Read the model definition and answer for the solid it produces. Units are mm, in the model's axes. Face numbers are marked on the shaded views. A direction names the side the tool comes from. Coordinates: 2 decimals unless noted, no trailing zeros. Write each loop counter-clockwise with the first axis right and the second up, starting at its lowest first coordinate (ties: lowest second). Pieces come first, ordered by that corner, then holes.
from build123d import *

# Parameters (mm, degrees)
CROQUIS1_R              = 11
CROQUIS3_R              = 11.5
CROQUIS4_R              = 7.5
CROQUIS5_R              = 8
CROQUIS6_R              = 16
CROQUIS6_R_2            = 8
SALIENTE_EXTRUIR1_DEPTH = 2


with BuildPart() as part:
    # Croquis1 → Recubrir1 section 0
    with BuildSketch(Plane.XY):
        Circle(CROQUIS1_R)
    # Croquis3 → Recubrir1 section 1
    with BuildSketch(Plane.XY.offset(33)):
        Circle(CROQUIS3_R)
    loft()

    # Croquis4 → Cortar-Recubrir1 section 0
    with BuildSketch(Plane(origin=(0, 0, 0), x_dir=(-1, 0, 0), z_dir=(0, 0, -1))):
        Circle(CROQUIS4_R)
    # Croquis5 → Cortar-Recubrir1 section 1
    with BuildSketch(Plane.XY.offset(33)):
        Circle(CROQUIS5_R)
    loft(mode=Mode.SUBTRACT)

    # Croquis6 → Saliente-Extruir1 (add)
    with BuildSketch(Plane.XY.offset(33)):
        Circle(CROQUIS6_R)
        Circle(CROQUIS6_R_2, mode=Mode.SUBTRACT)
    extrude(amount=SALIENTE_EXTRUIR1_DEPTH)


solid = part.part
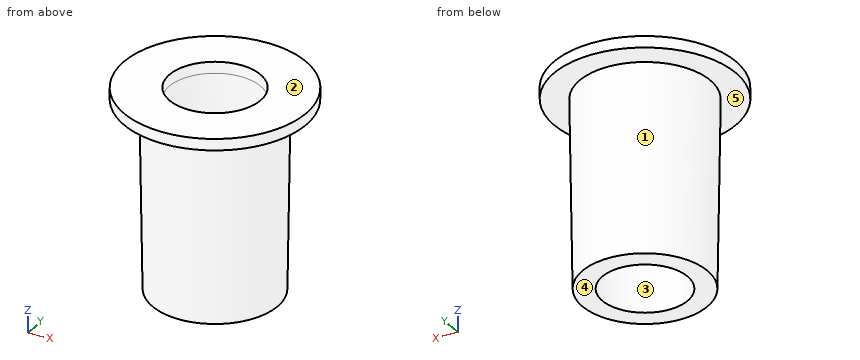
Item 1: The part is cut by section A-A (z = 14). Give the vertices of the cut face in (x, y).
Item 2: Find the intervals of material crossed by probe 1 along Y at (x, z) = (0, 34.5); probe 2 along Y at (x, z) = (-7, 25); probe 3 along X at (y, z) = (6, 10.5), in increasing order.
Item 3: Given pin 1 (2 mm diameter, centred on y = 12.5, z = 20.5, fed in from -X); pin 2 (5 mm diameter, centred on y = 7, z = 15, fed in from -X); pin 3 (4 mm diameter, centred on y = -10.5, z = 18, fed in from +X), each flat-ended and moving along its own axis, determine where each tip first touches the part or whether it passes through.
Item 4: For the marked faces 4 and 5, determine the directions among +Z, -Z, +X, -X, +Y, -Y from which every point of the face is accessible in a straight line to the end or side of a thin tool.
Item 5: The part is cut by section C-C (z = 9.5). Give the vertices of the cut face in (x, y).
Item 6: Determine the mould class of the marked faces 1, 2 and 3 for opening direction X: +X half, -X half, draft (parallel to the pull), parting line (faces both ways), or undercut.
Item 7: The part is cut by section B-B (x = 13.5). Give the vertices of the cut face in (y, z).
Answer:
1. outline: circle Ø22.42 at (0, 0); hole circle Ø15.42 at (0, 0)
2. probe 1: y = -16 to -8, 8 to 16
2. probe 2: y = -8.97 to -3.62, 3.62 to 8.97
2. probe 3: x = -9.41 to -4.76, 4.76 to 9.41
3. pin 1: passes through
3. pin 2: stops at x = -10.29
3. pin 3: stops at x = 7.4
4. face 4: -Z, +X, -X, +Y, -Y
4. face 5: -Z
5. outline: circle Ø22.29 at (0, 0); hole circle Ø15.29 at (0, 0)
6. face 1: parting line
6. face 2: draft
6. face 3: undercut
7. outline: (-8.59, 33) - (8.59, 33) - (8.59, 35) - (-8.59, 35) - close
